```python
from build123d import *

# Parameters (mm, degrees)
BOSS_EXTRUDE2_DEPTH = 300
CUT_EXTRUDE1_DEPTH  = 100


with BuildPart() as part:
    # Sketch1 → Boss-Extrude2 (new body)
    with BuildSketch(Plane.XY):
        with BuildLine():
            Line((0, 0), (-11.7, 0))
            ThreePointArc((-11.7, 0), (-12.972792206, 0.527207794), (-13.5, 1.8))
            Line((-13.5, 1.8), (-13.5, 6.7))
            ThreePointArc((-13.5, 6.7), (-13.734314575, 7.265685425), (-14.3, 7.5))
            Line((-14.3, 7.5), (-17.5, 7.5))
            Line((-17.5, 7.5), (-17.5, 8.5))
            Line((-17.5, 8.5), (-14.3, 8.5))
            ThreePointArc((-14.3, 8.5), (-13.027207794, 7.972792206), (-12.5, 6.7))
            Line((-12.5, 6.7), (-12.5, 1.8))
            ThreePointArc((-12.5, 1.8), (-12.265685425, 1.234314575), (-11.7, 1))
            Line((-11.7, 1), (0, 1))
            Line((0, 1), (11.7, 1))
            ThreePointArc((11.7, 1), (12.265685425, 1.234314575), (12.5, 1.8))
            Line((12.5, 1.8), (12.5, 6.7))
            ThreePointArc((12.5, 6.7), (13.027207794, 7.972792206), (14.3, 8.5))
            Line((14.3, 8.5), (17.5, 8.5))
            Line((17.5, 8.5), (17.5, 7.5))
            Line((17.5, 7.5), (14.3, 7.5))
            ThreePointArc((14.3, 7.5), (13.734314575, 7.265685425), (13.5, 6.7))
            Line((13.5, 6.7), (13.5, 1.8))
            ThreePointArc((13.5, 1.8), (12.972792206, 0.527207794), (11.7, 0))
            Line((11.7, 0), (0, 0))
        make_face()
    extrude(amount=BOSS_EXTRUDE2_DEPTH)

    # Sketch2 → Cut-Extrude1 (cut)
    with BuildSketch(Plane(origin=(0, 1, 0), x_dir=(1, 0, 0), z_dir=(0, 1, 0))):
        with BuildLine():
            Line((-3.1, -290), (-3.1, -275))
            ThreePointArc((-3.1, -275), (0, -271.9), (3.1, -275))
            Line((3.1, -275), (3.1, -290))
            ThreePointArc((3.1, -290), (0, -293.1), (-3.1, -290))
        make_face()
        with BuildLine():
            Line((-3.1, -265), (-3.1, -250))
            ThreePointArc((-3.1, -250), (0, -246.9), (3.1, -250))
            Line((3.1, -250), (3.1, -265))
            ThreePointArc((3.1, -265), (0, -268.1), (-3.1, -265))
        make_face()
        with BuildLine():
            Line((-3.1, -240), (-3.1, -225))
            ThreePointArc((-3.1, -225), (0, -221.9), (3.1, -225))
            Line((3.1, -225), (3.1, -240))
            ThreePointArc((3.1, -240), (0, -243.1), (-3.1, -240))
        make_face()
        with BuildLine():
            Line((-3.1, -215), (-3.1, -200))
            ThreePointArc((-3.1, -200), (0, -196.9), (3.1, -200))
            Line((3.1, -200), (3.1, -215))
            ThreePointArc((3.1, -215), (0, -218.1), (-3.1, -215))
        make_face()
        with BuildLine():
            Line((-3.1, -315), (-3.1, -300))
            ThreePointArc((-3.1, -300), (0, -296.9), (3.1, -300))
            Line((3.1, -300), (3.1, -315))
            ThreePointArc((3.1, -315), (0, -318.1), (-3.1, -315))
        make_face()
        with BuildLine():
            Line((-3.1, -190), (-3.1, -175))
            ThreePointArc((-3.1, -175), (0, -171.9), (3.1, -175))
            Line((3.1, -175), (3.1, -190))
            ThreePointArc((3.1, -190), (0, -193.1), (-3.1, -190))
        make_face()
        with BuildLine():
            Line((-3.1, -165), (-3.1, -150))
            ThreePointArc((-3.1, -150), (0, -146.9), (3.1, -150))
            Line((3.1, -150), (3.1, -165))
            ThreePointArc((3.1, -165), (0, -168.1), (-3.1, -165))
        make_face()
        with BuildLine():
            Line((-3.1, -140), (-3.1, -125))
            ThreePointArc((-3.1, -125), (0, -121.9), (3.1, -125))
            Line((3.1, -125), (3.1, -140))
            ThreePointArc((3.1, -140), (0, -143.1), (-3.1, -140))
        make_face()
        with BuildLine():
            Line((-3.1, -115), (-3.1, -100))
            ThreePointArc((-3.1, -100), (0, -96.9), (3.1, -100))
            Line((3.1, -100), (3.1, -115))
            ThreePointArc((3.1, -115), (0, -118.1), (-3.1, -115))
        make_face()
        with BuildLine():
            Line((-3.1, -90), (-3.1, -75))
            ThreePointArc((-3.1, -75), (0, -71.9), (3.1, -75))
            Line((3.1, -75), (3.1, -90))
            ThreePointArc((3.1, -90), (0, -93.1), (-3.1, -90))
        make_face()
        with BuildLine():
            Line((-3.1, -65), (-3.1, -50))
            ThreePointArc((-3.1, -50), (0, -46.9), (3.1, -50))
            Line((3.1, -50), (3.1, -65))
            ThreePointArc((3.1, -65), (0, -68.1), (-3.1, -65))
        make_face()
        with BuildLine():
            Line((-3.1, -40), (-3.1, -25))
            ThreePointArc((-3.1, -25), (0, -21.9), (3.1, -25))
            Line((3.1, -25), (3.1, -40))
            ThreePointArc((3.1, -40), (0, -43.1), (-3.1, -40))
        make_face()
        with BuildLine():
            Line((-3.1, -15), (-3.1, 0))
            ThreePointArc((-3.1, 0), (0, 3.1), (3.1, 0))
            Line((3.1, 0), (3.1, -15))
            ThreePointArc((3.1, -15), (0, -18.1), (-3.1, -15))
        make_face()
    extrude(amount=-CUT_EXTRUDE1_DEPTH, mode=Mode.SUBTRACT)


solid = part.part
```
Could you check a few things on this model? Use its own coordinates, in mm. A direction names the side the tool comes from. Round coordinates to 2 decimals unless told otherwise and drop trailing zeros. Loops run counter-clockwise (first coordinate to the right, second up) from the corner with the lowest first, then second, coordinate; pieces in that order, holes last. Notation, with made-up numbers: M 66,-39.75 L 84,-39.75 A27 cw 84,-12.75 Z; hole C 3.25,15.25 d8. An arc over 180 degrees is marked long. Write item = value, one per line.
1. I want a section at B-B, the plane y = 3.25. Write out the boundary of the cut face in (x, z).
Results below:
outline = M -13.5,0 L -12.5,0 L -12.5,300 L -13.5,300 Z; M 12.5,0 L 13.5,0 L 13.5,300 L 12.5,300 Z
2. Which directions (+Z, -Z, +X, -X, +Y, -Y) give clear straight access to the entire face, cutting with the end or side of a thin tool? Please do faces 1 (the face through (-3, 1, 148)), 2 (the face through (13, 3, 0)), 3 (the face through (-13.5, 4, 148)).
Results below:
face_1 = +Z, -Z, +Y
face_2 = -Z, +X, -X, +Y, -Y
face_3 = +Z, -Z, -X, -Y
3. Thinking about a two-plate mould opening in X: for faces 4 (the face through (-12.5, 4, 148)), 5 (the face through (13.5, 4, 148)), 6 (the face through (-13, 3, 300)), 7 (the face through (12.5, 4, 148)), which applies, +X half, -X half, draft (parallel to the pull), parting line (faces both ways), or undercut?
Results below:
face_4 = undercut
face_5 = +X half
face_6 = draft
face_7 = undercut
4. Will these pins go through, and if not, where does the flat tip stop? P1, Ø0.8, axis at y = 0.5, z = 7, coming from the -X side; P2, Ø6, axis at x = -4.5, z = 76, coming from the +Y side; P3, Ø0.5, axis at y = 0.5, z = 259, coming from the -X side.
Results below:
P1 = -13.26
P2 = 1
P3 = -13.16
5. I want a section at C-C, the plane x = 9. Write out the boundary of the cut face in (y, z).
Results below:
outline = M 0,0 L 1,0 L 1,300 L 0,300 Z
6. I need wall thicknesses on probe 1 along X at (y, z) = (1.5, 171); probe 2 along X at (y, z) = (4.75, 130); probe 3 along Y at (x, z) = (-0.5, 246.5). Which ranges of each line are inside material? Lowest first, please.
Results below:
probe_1 = -13.47 to -12.44, 12.44 to 13.47
probe_2 = -13.5 to -12.5, 12.5 to 13.5
probe_3 = 0 to 1
7. I want a section at A-A, the plane z = 155. Write out the boundary of the cut face in (x, y), and give its area (3 significant figures).
Results below:
outline = M -17.5,7.5 L -14.3,7.5 A0.8 cw -13.5,6.7 L -13.5,1.8 A1.8 ccw -11.7,0 L -3.1,0 L -3.1,1 L -11.7,1 A0.8 cw -12.5,1.8 L -12.5,6.7 A1.8 ccw -14.3,8.5 L -17.5,8.5 Z; M 3.1,0 L 11.7,0 A1.8 ccw 13.5,1.8 L 13.5,6.7 A0.8 cw 14.3,7.5 L 17.5,7.5 L 17.5,8.5 L 14.3,8.5 A1.8 ccw 12.5,6.7 L 12.5,1.8 A0.8 cw 11.7,1 L 3.1,1 Z
area = 41.6 mm²
